Source: CAD feature listing. Evaluate the final solid. Frame: model axes, mm. Coordinates: 2 decimals unless noted, no trailing zeros. Order: outer loops, then holes, each group sorted by start corner. A loop starts at its lowest first (then second) coordinate and runs counter-clockwise, first axis right, second up. Notation, with made-up numbers: (32.25, 33.5) - (74.25, 33.5) arc R25 cw to (74.25, 65.5) - close; hole circle Ø5 at (41, -19.5). An arc over 180 degrees is marked (long way). One line per question, with ' | ' between items.
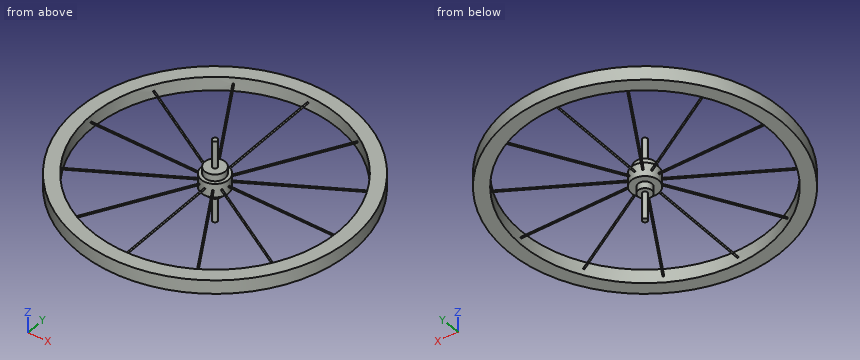
from build123d import *

# Parameters (mm, degrees)
BOSS_EXTRUDE1_DEPTH      = 12.7
BOSS_EXTRUDE1_DEPTH_BACK = 12.7
SKETCH1_R                = 25.4
SWEEP1_PROFILE_R         = 1.27
CIRPATTERN1_COUNT        = 12
BOSS_EXTRUDE2_DEPTH      = 12.7
BOSS_EXTRUDE2_DEPTH_BACK = 12.7
SKETCH43_R               = 254
SKETCH43_R_2             = 228.6
SKETCH44_R               = 19.05
BOSS_EXTRUDE3_DEPTH      = 12.7
SKETCH46_R               = 12.7
BOSS_EXTRUDE4_DEPTH      = 12.7
BOSS_EXTRUDE5_DEPTH      = 76.2
BOSS_EXTRUDE5_DEPTH_BACK = 76.2
SKETCH47_R               = 4.7625


with BuildPart() as part:
    # Sketch1 → Boss-Extrude1 (new, two sides: drawn at the far end of the back side and taken through both)
    with BuildSketch(Plane.XY.offset(-BOSS_EXTRUDE1_DEPTH_BACK)):
        Circle(SKETCH1_R)
    extrude(amount=BOSS_EXTRUDE1_DEPTH + BOSS_EXTRUDE1_DEPTH_BACK)

    # Sweep1: sweep along a path in Sketch2
    with BuildLine(Plane.XY) as sweep1_path:
        Line((0, 0), (228.6, 0))
    # Sweep1 profile (on start of the path) → Sweep1 (sweep)
    with BuildSketch(Plane(origin=(0, 0, 0), x_dir=(0, 0, 1), z_dir=(1, 0, 0))):
        Circle(SWEEP1_PROFILE_R)
    sweep1 = sweep(path=sweep1_path.line)

    # CirPattern1: Sweep1 ×12 about axis
    cirpattern1_axis = Axis((0, 0, 0), (0, 0, 1))
    for i in range(1, CIRPATTERN1_COUNT):
        add(sweep1.rotate(cirpattern1_axis, i * 360 / CIRPATTERN1_COUNT))

    # Sketch43 → Boss-Extrude2 (add, two sides: drawn at the far end of the back side and taken through both)
    with BuildSketch(Plane.XY.offset(-BOSS_EXTRUDE2_DEPTH_BACK)):
        Circle(SKETCH43_R)
        Circle(SKETCH43_R_2, mode=Mode.SUBTRACT)
    extrude(amount=BOSS_EXTRUDE2_DEPTH + BOSS_EXTRUDE2_DEPTH_BACK)

    # Sketch44 → Boss-Extrude3 (add)
    with BuildSketch(Plane.XY.offset(12.7)):
        Circle(SKETCH44_R)
    extrude(amount=BOSS_EXTRUDE3_DEPTH)

    # Sketch46 → Boss-Extrude4 (add)
    with BuildSketch(Plane(origin=(0, 0, -12.7), x_dir=(-1, 0, 0), z_dir=(0, 0, -1))):
        with Locations(Location((0, 0, 0), (0, 0, 180))):
            Circle(SKETCH46_R)
    extrude(amount=BOSS_EXTRUDE4_DEPTH)

    # Sketch47 → Boss-Extrude5 (add, two sides: drawn at the far end of the back side and taken through both)
    with BuildSketch(Plane.XY.offset(-BOSS_EXTRUDE5_DEPTH_BACK)):
        Circle(SKETCH47_R)
    extrude(amount=BOSS_EXTRUDE5_DEPTH + BOSS_EXTRUDE5_DEPTH_BACK)


solid = part.part
(1) Material intervals for L1, parallel to Y at x = 0, z = 3.25; L2, parallel to Y at x = -121, z = -10; L3, parallel to Z at x = -225.5, y = -81.5, sorted ascending. Write a range as from..to.
Taken from the geometry:
L1: y = -254..-228.6, -25.4..25.4, 228.6..254 | L2: y = -223.33..-193.95, 193.95..223.33 | L3: z = -12.7..12.7
(2) Pin query (flat end, axial travel): P1, Ø15, axis at x = -11.5, y = 5.5, coming from the -Z side; P2, Ø6, axis at x = -168.5, y = 97.5, coming from the +Z side; P3, Ø12, axis at y = -153, z = 1.5, coming from the +X side. Return the tip coordinate at first contact, or that it passes through.
Taken from the geometry:
P1: stops at z = -25.4 | P2: stops at z = 1.27 | P3: stops at x = 207.14
(3) Cut plane A-A (x = 221). Return the cut outline in (y, z).
Taken from the geometry:
outline: (-125.2, -12.7) - (-58.45, -12.7) - (-58.45, 12.7) - (-125.2, 12.7) - close; circle Ø2.54 at (0, 0); (58.45, -12.7) - (125.2, -12.7) - (125.2, 12.7) - (58.45, 12.7) - close
(4) Cut plane B-B (y = -96). State how many separate pieces and enclosed holes the cut face has, and give its area (3 significant figures).
Taken from the geometry:
separate pieces: 7 | enclosed holes: 0 | area: 1,440 mm²
